from build123d import *

# Parameters (mm, degrees)
BOX001_W        = 0.63
BOX001_H        = 0.63
BOX001_DEPTH    = 17
CHAMFER001_SIZE = 0.3
BOX_W           = 2.54
BOX_H           = 2.54
BOX_DEPTH       = 2.8
CHAMFER_SIZE    = 0.25


with BuildPart() as pin:
    # Box001 → Box001 (new body)
    with BuildSketch(Plane(origin=(-3, 0, 0), x_dir=(1, 0, 0), z_dir=(0, 0, 1))):
        with Locations((0.315, 0.315)):
            Rectangle(BOX001_W, BOX001_H)
    extrude(amount=BOX001_DEPTH)

    # Chamfer001
    chamfer001_edges = [pin.edges().sort_by_distance(p)[0] for p in [
        (-3, 0.315, 17),
        (-3, 0.315, 0),
        (-2.37, 0.315, 17),
        (-2.37, 0.315, 0),
        (-2.685, 0, 0),
        (-2.685, 0, 17),
        (-2.685, 0.63, 0),
        (-2.685, 0.63, 17),
    ]]
    chamfer(chamfer001_edges, length=CHAMFER001_SIZE)


with BuildPart() as pin_1:
    # Chamfer001 placement: moved
    add(pin.part.moved(Location((3.95, 0.95, -6))))


with BuildPart() as single_pin:
    # Box → Box (new body)
    with BuildSketch(Plane.XY):
        with Locations((1.27, 1.27)):
            Rectangle(BOX_W, BOX_H)
    extrude(amount=BOX_DEPTH)

    # Chamfer
    chamfer_edges = [single_pin.edges().sort_by_distance(p)[0] for p in [
        (0, 0, 1.4),
        (0, 1.27, 2.8),
        (0, 2.54, 1.4),
        (0, 1.27, 0),
        (2.54, 0, 1.4),
        (2.54, 1.27, 2.8),
        (2.54, 2.54, 1.4),
        (2.54, 1.27, 0),
        (1.27, 0, 0),
        (1.27, 0, 2.8),
        (1.27, 2.54, 0),
        (1.27, 2.54, 2.8),
    ]]
    chamfer(chamfer_edges, length=CHAMFER_SIZE)

    # Fusion: union Pin
    add(pin_1.part)


solid = single_pin.part
CAD build for the part. Positions are in the model's coordinates, mm. Coordinates: 2 decimals unless noted, no trailing zeros. Loops run counter-clockwise (first coordinate to the right, second up) from the corner with the lowest first, then second, coordinate; pieces in that order, holes last. Notation, with made-up numbers: (86.25, 47.25) - (109.25, 47.25) arc R21 ccw to (109.25, 69.25) - close; hole circle Ø10 at (88.25, 71). An arc over 180 degrees is marked (long way). Write item = value, one per line. Start each with the question number.
Q1. Cut at C-C, the plane z = 8.5. List the corners of the cut face in (x, y), then the cut area to 3 significant figures.
Q2. Cut at B-B, the plane z = 1.25. List the corners of the cut face in (x, y).
Q3. Drill centre lines: L1, parallel to Z at x = 1.7, y = 1.8; L2, parallel to Y at x = 1.4, z = 6.25; L3, parallel to Z at x = 2.35, y = 1.55. Where is each one in solid material? Low to high.
Q4. Cut at A-A, the plane x = 0.7. List the corners of the cut face in (y, z), then the cut area to 3 significant figures.
Q5. Flat gauge pins, fed straight in: pin 1 Ø0.5 at (x, z) = (1.5, 6) entering from -Y; pin 2 Ø0.5 at (x, z) = (1.5, -3.5) entering from +Y; pin 3 Ø0.7 at (y, z) = (1, 8) entering from +X. Where does each tip first touch, or does it go through?
Computed:
q1.outline = (0.95, 0.95) - (1.58, 0.95) - (1.58, 1.58) - (0.95, 1.58) - close
q1.area = 0.397 mm²
q2.outline = (0, 0.25) - (0.25, 0) - (2.29, 0) - (2.54, 0.25) - (2.54, 2.29) - (2.29, 2.54) - (0.25, 2.54) - (0, 2.29) - close
q3.L1 = 0 to 2.8
q3.L2 = 0.95 to 1.58
q3.L3 = 0.06 to 2.74
q4.outline = (0, 0.25) - (0.25, 0) - (2.29, 0) - (2.54, 0.25) - (2.54, 2.55) - (2.29, 2.8) - (0.25, 2.8) - (0, 2.55) - close
q4.area = 6.99 mm²
q5.pin_1 = 0.95
q5.pin_2 = 1.58
q5.pin_3 = 1.58
